Could you check a few things on this model? Use its own coordinates, in mm. Face numbers are marked on the shaded views. A direction names the side the tool comes from. Round coordinates to 2 decimals unless told otherwise and drop trailing zeros. Order: outer loops, then holes, each group sorted by start corner. A loop starts at its lowest first (then second) coordinate and runs counter-clockwise, first axis right, second up.
Autodesk Inventor part; units mm, degrees
ref_plane "YZ Plane" through (0, 0, 0) normal (1, 0, 0) x (0, 1, 0)
ref_plane "XZ Plane" through (0, 0, 0) normal (0, 1, 0) x (-1, 0, 0)
ref_plane "XY Plane" through (0, 0, 0) normal (0, 0, 1) x (1, 0, 0)
sketch "スケッチ1" plane through (0, 0, 0) normal (0, 0, 1) x (1, 0, 0)
  line L0 (-20, 25) -> (20, 25)
  line L1 (20, 25) -> (20, -25)
  line L2 (20, -25) -> (-20, -25)
  line L3 (-20, -25) -> (-20, 25)
  point P0 (0, 0)
  dimension "d0" = 50
  dimension "d1" = 40
  dimension "d2" = 20
  dimension "d3" = 25
extrude "押し出し1" add sketch "スケッチ1" along normal blind 5
sketch "スケッチ2" plane through (0, 0, 5) normal (0, 0, 1) x (1, 0, 0)
  line L0 (20, 25) -> (20, -25)
  line L1 (-20, -25) -> (-20, 25)
  line L2 (20, -25) -> (-20, -25)
  line L3 (-20, 25) -> (20, 25)
  line L4 (20, 25) -> (20, 19.9)
  line L5 (20, 19.9) -> (-20, 19.9)
  line L6 (-20, 19.9) -> (-20, 25)
  line L7 (20, -25) -> (-20, -25)
  line L8 (-20, -25) -> (-20, -19.9)
  line L9 (-20, -19.9) -> (20, -19.9)
  line L10 (20, -19.9) -> (20, -25)
  point P0 (0, 0)
  dimension "d6" = 5.1
  dimension "d7" = 5.1
  dimension "d12" = 0
extrude "押し出し3" cut sketch "スケッチ2" against normal blind 2 contours L0 L5 L1 L3 | L0 L2 L1 L9
sketch "スケッチ3" plane through (0, 0, 5) normal (0, 0, 1) x (1, 0, 0)
  point P0 (0, 0)
  point P1 (0, 10)
  point P2 (0, -10)
  dimension "d13" = 20
  dimension "d14" = 10
hole "Hole1" at (0, 10, 5) at (0, -10, 5) direction (0, 0, -1) diameter 6 end through all
sketch "スケッチ4" plane through (0, 0, 0) normal (0, 0, -1) x (-1, 0, 0)
  circle A0 centre (0, -10) radius 3
  circle A1 centre (0, 10) radius 3
  line L0 (20, 25) -> (-20, 25)
  line L1 (-20, 25) -> (-13.5, 25)
  line L2 (-13.5, 25) -> (-13.5, 19.9)
  line L3 (-13.5, 19.9) -> (-20, 19.9)
  line L4 (-20, 19.9) -> (-20, 25)
  line L5 (20, 25) -> (13.5, 25)
  line L6 (13.5, 25) -> (13.5, 19.9)
  line L7 (13.5, 19.9) -> (20, 19.9)
  line L8 (20, 19.9) -> (20, 25)
  line L9 (20, -25) -> (13.5, -25)
  line L10 (13.5, -25) -> (13.5, -19.9)
  line L11 (13.5, -19.9) -> (20, -19.9)
  line L12 (20, -19.9) -> (20, -25)
  line L13 (-20, -25) -> (-13.5, -25)
  line L14 (-13.5, -25) -> (-13.5, -19.9)
  line L15 (-13.5, -19.9) -> (-20, -19.9)
  line L16 (-20, -19.9) -> (-20, -25)
  point P0 (0, 0)
  dimension "d22" = 5.1
  dimension "d23" = 5.1
  dimension "d24" = 5.1
  dimension "d25" = 5.1
  dimension "d26" = 27
  dimension "d27" = 13.5
  dimension "d28" = 13.5
  dimension "d29" = 27
extrude "押し出し4" cut sketch "スケッチ4" against normal through all contours L8 L7 L6 L0 | L2 L3 L4 L0 | L9 L10 L11 L12 | L16 L15 L14 L13
sketch "スケッチ5" plane through (0, 0, 5) normal (0, 0, 1) x (1, 0, 0)
  line L0 (20, 19.9) -> (-20, 19.9)
  line L1 (-20, -19.9) -> (-20, 19.9)
  line L2 (-20, -19.9) -> (20, -19.9)
  line L3 (20, 19.9) -> (20, -19.9)
  point P0 (0, 0)
  point P1 (-14, 13.9)
  point P2 (-14, -13.9)
  point P3 (14, -13.9)
  point P4 (14, 13.9)
  dimension "d32" = 6
  dimension "d33" = 6
  dimension "d34" = 6
  dimension "d35" = 6
  dimension "d36" = 6
  dimension "d37" = 6
  dimension "d38" = 6
  dimension "d39" = 6
hole "Hole2" at (-14, 13.9, 5) at (-14, -13.9, 5) at (14, -13.9, 5) at (14, 13.9, 5) direction (0, 0, -1) diameter 2.8 depth 8 tip angle 118
sketch "スケッチ6" plane through (0, 0, 0) normal (0, 0, -1) x (-1, 0, 0)
  line L0 (-20, -19.9) -> (-13.5, -19.9)
  line L1 (-13.5, -19.9) -> (-13.5, -25)
  line L2 (13.5, -25) -> (13.5, -19.9)
  line L3 (13.5, -19.9) -> (20, -19.9)
  line L4 (20, 19.9) -> (13.5, 19.9)
  line L5 (13.5, 19.9) -> (13.5, 25)
  line L6 (-13.5, 19.9) -> (-20, 19.9)
  line L7 (-13.5, 19.9) -> (-13.5, 25)
  point P0 (0, 0)
  point P1 (-13.5, 20.9)
  point P2 (13.5, 20.9)
  point P3 (13.5, -20.9)
  point P4 (-13.5, -20.9)
  dimension "d47" = 1
  dimension "d48" = 1
  dimension "d49" = 1
  dimension "d50" = 1
hole "Hole3" at (13.5, 20.9, 0) at (-13.5, 20.9, 0) at (-13.5, -20.9, 0) at (13.5, -20.9, 0) direction (0, 0, 1) diameter 2 depth 8 tip angle 118
equation "\"d23\" = d22"
equation "\"d24\" = d22"
equation "\"d25\" = d22"
equation "\"d27\" = 0.5 * d26"
equation "\"d28\" = d27"
equation "\"d29\" = d26"
properties part number "JointC0_"
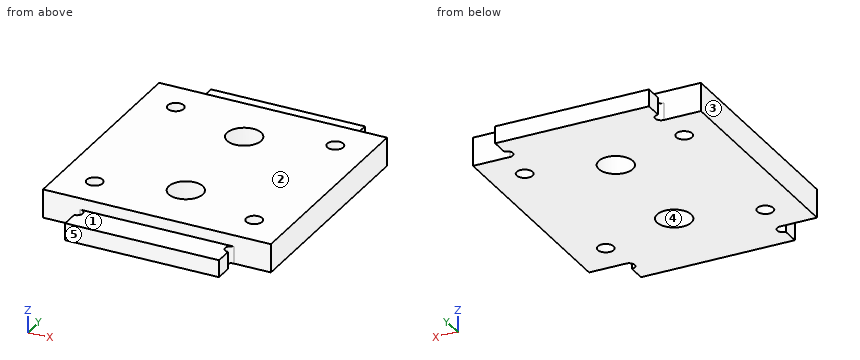
Q1. I need wall thicknesses on L1, parallel to X at y = -13.9, z = 3.9; L2, parallel to Y at x = 0, z = 2.3; L3, parallel to Y at x = 14, z = 2.95. Which ranges of each line are inside material? Lowest first, please.
Q2. For the marked faces 1 and 2, which set-ups out of +Z, -Z, +X, -X, +Y, -Y let a thin tool reach every point of the face, with its end or its side?
Q3. Imagine slicing it at A-A, the plane z = 2.05. Please give me the cut outline in (x, y), then the cut area to 3 significant figures.
Q4. Imagine slicing it at D-D, the plane x = -16. Please give me the cut outline in (y, z), then the cut area to 3 significant figures.
Q5. For P1, Ø3.5, axis at x = 14, y = 13.9, coming from the -Z side; P2, Ø4, axis at x = 0.5, y = -23, coming from the +Z side; P3, Ø1.5, axis at y = -23.5, z = 1, coming from the -X side; P4, Ø1.5, axis at y = 22.5, z = 1.5, coming from the +X side, each with a flat end and sliding along its axis, tell me the tip position at first contact or that it passes through.
Q6. Imagine slicing it at B-B, the plane x = 0. Please give me the cut outline in (y, z), then the cut area to 3 significant figures.
Q7. Imagine slicing it at C-C, the plane y = 13.9. Please give me the cut outline in (x, z), then the cut area to 3 significant figures.
Q8. We'd pull the mould along Y, two halves only. Please class the marked faces 3, 4 and 5: released by +Y, released by -Y, zero draft, split by the parting line, or undercut.
Filled in:
1. L1: x = -20 to -15.4, -12.6 to 12.6, 15.4 to 20
1. L2: y = -25 to -13, -7 to 7, 13 to 25
1. L3: y = -19.9 to -15.3, -12.5 to 12.5, 15.3 to 19.9
2. face 1: +Z, +X, -X, -Y
2. face 2: +Z, +X, -X, +Y, -Y
3. outline: (-20, -19.9) - (-13.5, -19.9) arc R1 cw to (-13.5, -21.9) - (-13.5, -25) - (13.5, -25) - (13.5, -21.9) arc R1 cw to (13.5, -19.9) - (20, -19.9) - (20, 19.9) - (13.5, 19.9) arc R1 cw to (13.5, 21.9) - (13.5, 25) - (-13.5, 25) - (-13.5, 21.9) arc R1 cw to (-13.5, 19.9) - (-20, 19.9) - close; hole circle Ø2.8 at (-14, -13.9); hole circle Ø2.8 at (-14, 13.9); hole circle Ø6 at (0, -10); hole circle Ø6 at (0, 10); hole circle Ø2.8 at (14, -13.9); hole circle Ø2.8 at (14, 13.9)
3. area: 1,780 mm2
4. outline: (-19.9, 0) - (19.9, 0) - (19.9, 5) - (-19.9, 5) - close
4. area: 199 mm2
5. P1: stops at z = 0
5. P2: stops at z = 3
5. P3: stops at x = -13.5
5. P4: stops at x = 13.5
6. outline: (-25, 0) - (-13, 0) - (-13, 5) - (-19.9, 5) - (-19.9, 3) - (-25, 3) - close; (-7, 0) - (7, 0) - (7, 5) - (-7, 5) - close; (13, 0) - (25, 0) - (25, 3) - (19.9, 3) - (19.9, 5) - (13, 5) - close
6. area: 170 mm2
7. outline: (-20, 0) - (-15.4, 0) - (-15.4, 5) - (-20, 5) - close; (-12.6, 0) - (12.6, 0) - (12.6, 5) - (-12.6, 5) - close; (15.4, 0) - (20, 0) - (20, 5) - (15.4, 5) - close
7. area: 172 mm2
8. face 3: zero draft
8. face 4: undercut
8. face 5: released by -Y
